from build123d import *

# Parameters (mm, degrees)
SKETCH1_W                           = 15.875
SKETCH1_H                           = 25.4
BOSS_EXTRUDE1_DEPTH                 = 50.8
TAP_DRILL_FOR_10_24_TAP1_D          = 3.7973
TAP_DRILL_FOR_10_24_TAP1_DEPTH      = 20.701
TAP_DRILL_FOR_10_24_TAP1_TIP        = 1.140824014
TAP_START                           = -25.4
TAP_DRILL_SLOT_FOR_10_24_TAP1_DEPTH = 25.4


# Read off the part's stored shape, not the designer's step: Tap Drill Slot for #10-24 Tap1
with BuildPart() as part:
    # Sketch1 → Boss-Extrude1 (new body)
    with BuildSketch(Plane(origin=(0, 0, 0), x_dir=(1, 0, 0), z_dir=(0, 1, 0))):
        with Locations((7.9375, 12.7)):
            Rectangle(SKETCH1_W, SKETCH1_H)
    extrude(amount=BOSS_EXTRUDE1_DEPTH)

    # Tap Drill for #10-24 Tap1
    with Locations(Plane(origin=(0, 0, 0), x_dir=(-1, 0, 0), z_dir=(0, -1, 0))):
        with Locations((-7.9375, 6), (-7.9375, 19.4)):
            Hole(TAP_DRILL_FOR_10_24_TAP1_D / 2, depth=TAP_DRILL_FOR_10_24_TAP1_DEPTH)
            with Locations((0, 0, -(TAP_DRILL_FOR_10_24_TAP1_DEPTH + TAP_DRILL_FOR_10_24_TAP1_TIP / 2))):  # 118° drill point
                Cone(0, TAP_DRILL_FOR_10_24_TAP1_D / 2, TAP_DRILL_FOR_10_24_TAP1_TIP, mode=Mode.SUBTRACT)

    # Tap Drill Slot for #10-24 Tap1 outline → Tap Drill Slot for #10-24 Tap1 (cut)
    with BuildSketch(Plane.XY.offset(TAP_START)):
        with BuildLine():
            Line((6.058801855, 24.6126), (9.868801855, 24.6126))
            ThreePointArc((9.868801855, 24.6126), (13.043801855, 27.7876), (9.868801855, 30.9626))
            Line((9.868801855, 30.9626), (6.058801855, 30.9626))
            ThreePointArc((6.058801855, 30.9626), (2.883801855, 27.7876), (6.058801855, 24.6126))
        make_face()
    extrude(amount=TAP_DRILL_SLOT_FOR_10_24_TAP1_DEPTH, mode=Mode.SUBTRACT)


solid = part.part
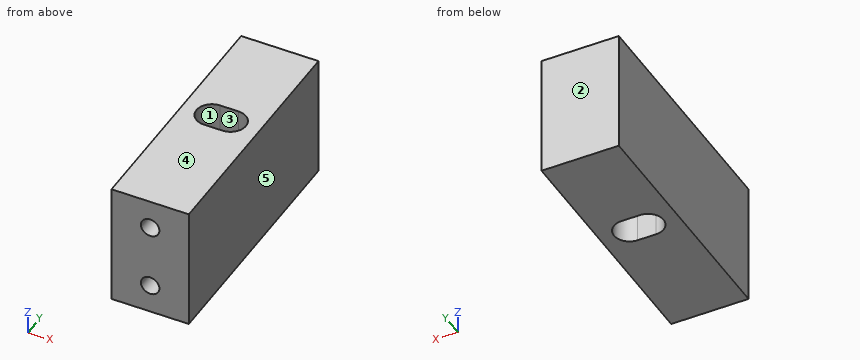
Geometry check sheet. Reference: the model listing, model coordinates, mm. Face numbers are marked on the shaded views. A direction names the side the tool comes from. Round coordinates to 2 decimals unless told otherwise and drop trailing zeros. Order: outer loops, then holes, each group sorted by start corner. A loop starts at its lowest first (then second) coordinate and runs counter-clockwise, first axis right, second up. Notation, with made-up numbers: M -7.75,21 L 30.25,21 A13 cw 30.25,27 Z; hole C 43.25,-29 d9. An arc over 180 degrees is marked long. Answer in a Markdown table with one row per item. Add a question column.
Item 1: Depth check by flat-ended pin: pin 1 Ø2.5 at (x, z) = (7.94, -19.4) entering from -Y. Enter the tip coordinate at first touch or a pass-through.
Item 2: Set-up check for the marked faces 1 and 2: record each of +Z, -Z, +X, -X, +Y, -Y from which the full face is reachable in a straight line by a thin tool's end or side.
Item 3: Material ranges on L1, parallel to Y at x = 7, z = -16; L2, parallel to X at y = 28, z = -19 (3 decimals); L3, parallel to X at y = 5.75, z = -19.4 (3 decimals), recorded low to high. Write a range as [from, to].
Item 4: Sectioned sample at A-A, the plane z = -15. Enter the section's corners in (x, y) (3 decimals).
Item 5: Draft check along X on the marked faces 3, 4 and 5. Enter one of: released by +X, released by -X, zero draft, split by the parting line, or undercut.
Filled in:
| question | item | result |
|---|---|---|
| 1 | pin 1 | stops at y = 21.09 |
| 2 | face 1 | +Z, -Z |
| 2 | face 2 | +Z, -Z, +X, -X, +Y |
| 3 | L1 | y = [0, 24.61], [30.96, 50.8] |
| 3 | L2 | x = [0, 2.891], [13.037, 15.875] |
| 3 | L3 | x = [0, 6.039], [9.836, 15.875] |
| 4 | outline | M 0,0 L 15.875,0 L 15.875,50.8 L 0,50.8 Z; hole M 6.059,24.613 L 9.869,24.613 A3.175 ccw 9.869,30.963 L 6.059,30.963 A3.175 ccw Z |
| 5 | face 3 | undercut |
| 5 | face 4 | zero draft |
| 5 | face 5 | released by +X |
